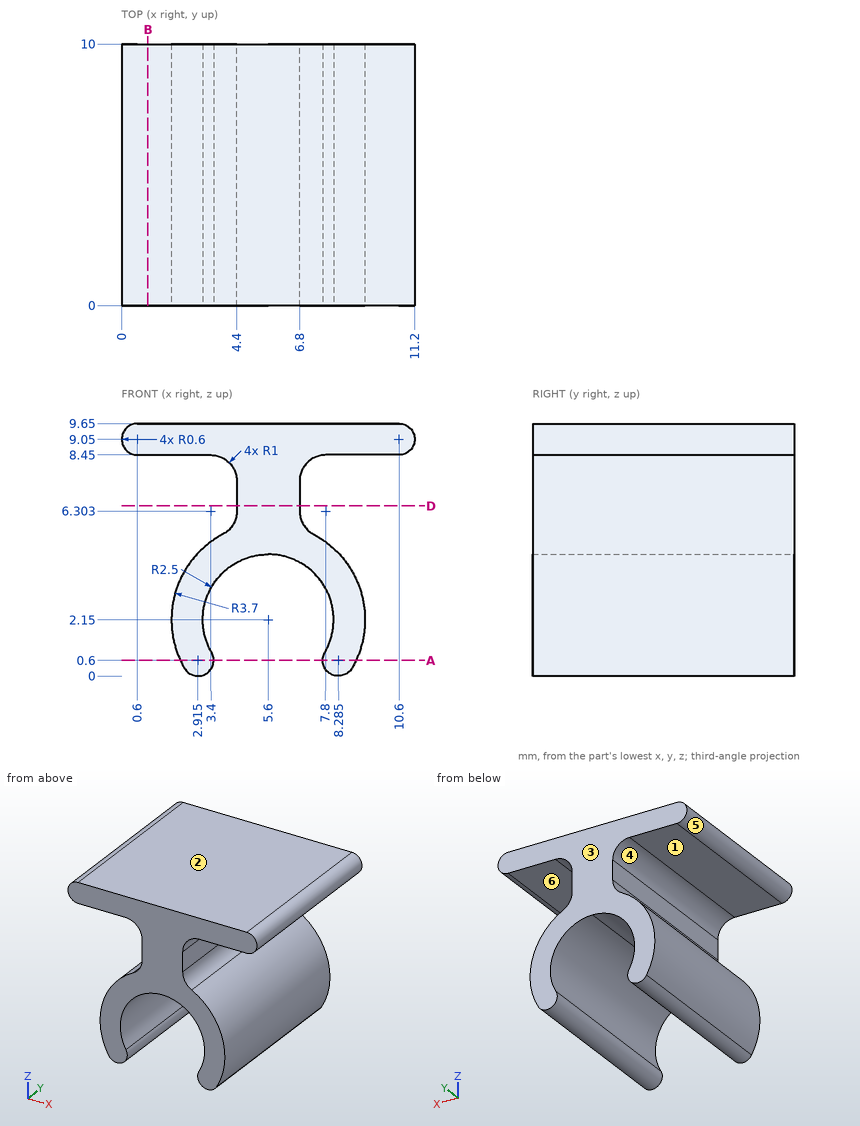
Check sheet for the drawn part. Datum: minimum x, y, z corner. Units: mm. A direction names the side the tool comes from. Give positions to 0.01 mm unless a question says otherwise; leave off trailing zeros. Write each loop counter-clockwise with the first axis right and the second up, starting at its lowest first coordinate (ties: lowest second). Pieces come first, ordered by that corner, then holes. Notation, with made-up numbers: M -1,-13.5 L 16,-13.5 A26 ccw 16,3.5 Z; hole C 60,6.25 d11. An arc over 180 degrees is marked long. One line per question, with ' | ' between items.
1. Cross-section at A-A (z = 0.6). Enter the section's corners in (x, y) (1 decimal).
Ans:
outline: M 2.2,0 L 3.5,0 L 3.5,10 L 2.2,10 Z; M 7.7,0 L 9,0 L 9,10 L 7.7,10 Z
2. Gauge pin test, flat ends, axial feed: pin 1 (1.5 mm diameter, centred on y = 3, z = 2.5, fed in from -X); pin 2 (1 mm diameter, centred on x = 9.5, y = 4.5, fed in from -Z); pin 3 (0.9 mm diameter, centred on y = 7, z = 7, fed in from +X). Record the tip position at first contact, or that the pin passes through.
Ans:
pin 1: x = 1.9 | pin 2: z = 0.69 | pin 3: x = 6.8
3. Scan lines: line 1 along X through (y, z) = (1.5, 7.5); line 2 along Z through (x, y) = (10, 6); line 3 along X through (y, z) = (4.5, 1.25). Record each from-to range of solid material in increasing order. Write a range as from..to.
Ans:
line 1: 4.4..6.8 | line 2: 8.45..9.65 | line 3: 2.01..3.27, 7.93..9.19
4. Mould release check, pull along Z, two halves, no side actions. Record for the marked faces 1, 2, 3 and 4: released by +Z, released by -Z, zero draft, split by the parting line, or undercut.
Ans:
face 1: undercut | face 2: released by +Z | face 3: zero draft | face 4: undercut
5. Cross-section at D-D (z = 6.5). Enter the section's corners in (x, y), plus the area to 3 significant figures.
Ans:
outline: M 4.4,0 L 6.8,0 L 6.8,10 L 4.4,10 Z | area: 24.0 mm2
6. Cross-section at B-B (x = 1). Enter the section's corners in (y, z).
Ans:
outline: M 0,8.45 L 10,8.45 L 10,9.65 L 0,9.65 Z
7. Set-up check for the marked faces 5 and 6: record each of +Z, -Z, +X, -X, +Y, -Y from which the full face is reachable in a straight line by a thin tool's end or side.
Ans:
face 5: -X, +Y, -Y | face 6: +X, +Y, -Y
